Design review of the part shown in the three views and the two pictorial views. Dimensions are in mm from the part's minimum x, y and z. A direction names the side the tool comes from. Round coordinates to 2 decimals unless told otherwise and drop trailing zeros. Loops run counter-clockwise (first coordinate to the right, second up) from the corner with the lowest first, then second, coordinate; pieces in that order, holes last.
1) Mouldability with a two-part tool opening along X and no side actions: class the marked faces 4, 5 and 6 as pulls with the +X half, pulls with the -X half, needs draft (parallel to the pull), parting line crosses it, or undercut.
2) Tool access review of the marked faces 1, 2 and 3: name each direction out of +Z, -Z, +X, -X, +Y, -Y from which nothing blocks a thin tool from reaching the whole face with its end or side.
3) Take a section at B-B (z = 8). State the section outline as (x, y) points, then the cut area to 3 significant figures.
4) Take a section at A-A (y = 3). State the section outline as (x, z) points.
5) Take a section at C-C (y = 22). State the section outline as (x, z) points.
6) Take a section at D-D (x = 23). State the section outline as (y, z) points, then the cut area to 3 significant figures.
7) Insertion check: pin 1 (4.5 mm diameter, centred on x = 21, y = 8.5, fed in from +Z); pin 2 (1 mm diameter, centred on y = 9, z = 4, fed in from -X); pin 3 (3 mm diameter, centred on x = 33, z = 23, fed in from +Y). Each pin has a flat end and moves straight along its axis. Give the tip position at first contact, or say it passes through.
8) Wall thickness on L1, parallel to Y at x = 44, z = 5.5; L2, parallel to X at y = 12, z = 25; L3, parallel to X at y = 8, z = 17.5: over which ranges is each line inside the solid? List them lowest first.
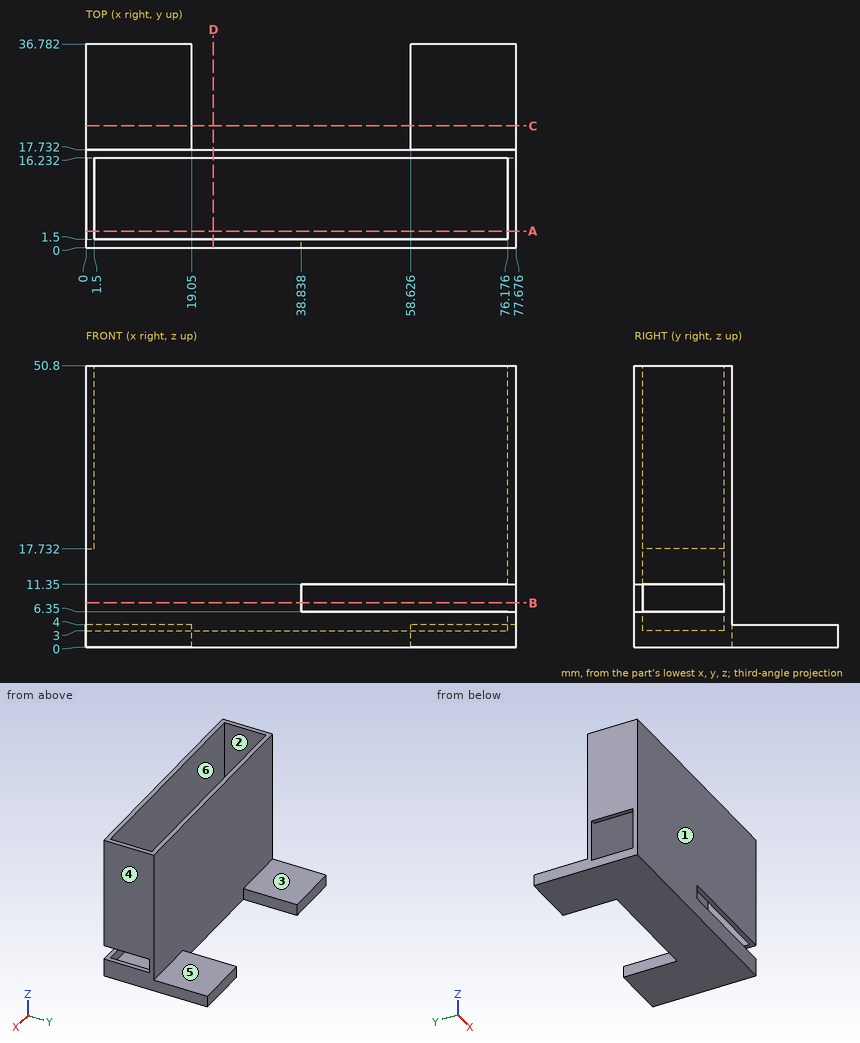
Response:
1. face 4: pulls with the +X half
1. face 5: needs draft
1. face 6: undercut
2. face 1: +Z, -Z, +X, -X, -Y
2. face 2: +Z
2. face 3: +Z, +X, -X, +Y
3. outline: (0, 0) - (38.84, 0) - (38.84, 1.5) - (0, 1.5) - close; (0, 16.23) - (77.68, 16.23) - (77.68, 17.73) - (0, 17.73) - close
3. area: 175 mm2
4. outline: (0, 0) - (77.68, 0) - (77.68, 6.35) - (76.18, 6.35) - (76.18, 3) - (0, 3) - close; (0, 17.73) - (1.5, 17.73) - (1.5, 50.8) - (0, 50.8) - close; (76.18, 11.35) - (77.68, 11.35) - (77.68, 50.8) - (76.18, 50.8) - close
5. outline: (0, 0) - (19.05, 0) - (19.05, 4) - (0, 4) - close; (58.63, 0) - (77.68, 0) - (77.68, 4) - (58.63, 4) - close
6. outline: (0, 0) - (17.73, 0) - (17.73, 50.8) - (16.23, 50.8) - (16.23, 3) - (1.5, 3) - (1.5, 50.8) - (0, 50.8) - close
6. area: 197 mm2
7. pin 1: stops at z = 3
7. pin 2: stops at x = 76.18
7. pin 3: stops at y = 17.73
8. L1: y = 0 to 1.5, 16.23 to 17.73
8. L2: x = 0 to 1.5, 76.18 to 77.68
8. L3: x = 76.18 to 77.68
